Part model, mm, in its own coordinate system. Face numbers are marked on the shaded views. A direction names the side the tool comes from. Coordinates: 2 decimals unless noted, no trailing zeros. Order: outer loops, then holes, each group sorted by start corner. A loop starts at its lowest first (then second) coordinate and runs counter-clockwise, first axis right, second up.
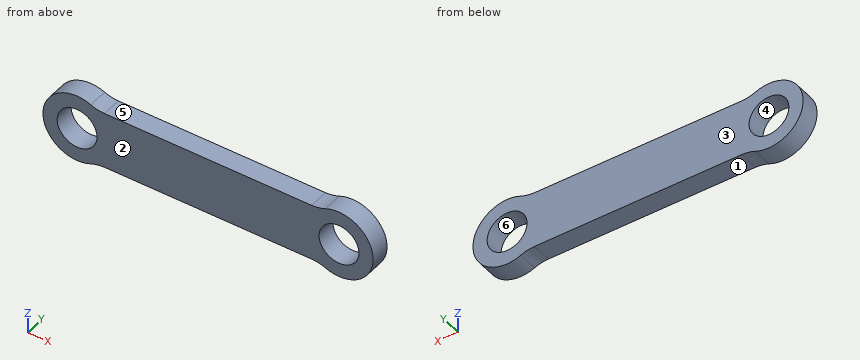
```python
from build123d import *

# Parameters (mm, degrees)
SKETCH1_R           = 1.75
BOSS_EXTRUDE1_DEPTH = 1.75
FILLET1_R           = 3


with BuildPart() as part:
    # Sketch1 → Boss-Extrude1 (new body)
    with BuildSketch(Plane(origin=(0, 0, 0), x_dir=(1, 0, 0), z_dir=(0, 1, 0))):
        with BuildLine():
            ThreePointArc((1.658312395, 2.5), (-3, 0), (1.658312395, -2.5))
            Line((1.658312395, -2.5), (21.341687605, -2.5))
            ThreePointArc((21.341687605, -2.5), (26, 0), (21.341687605, 2.5))
            Line((21.341687605, 2.5), (1.658312395, 2.5))
        make_face()
        with Locations(Location((0, 0, 0), (0, 0, 270))):
            Circle(SKETCH1_R, mode=Mode.SUBTRACT)
        with Locations(Location((23, 0, 0), (0, 0, 270))):
            Circle(SKETCH1_R, mode=Mode.SUBTRACT)
    extrude(amount=BOSS_EXTRUDE1_DEPTH)

    # Fillet1
    fillet1_edges = [part.edges().sort_by_distance(p)[0] for p in [
        (21.341687605, 0.875, 2.5),
        (1.658312395, 0.875, 2.5),
        (1.658312395, 0.875, -2.5),
        (21.341687605, 0.875, -2.5),
    ]]
    fillet(fillet1_edges, radius=FILLET1_R)


solid = part.part
```
(1) Tool access for the marked faces 1 and 2: list every direction of +Z, -Z, +X, -X, +Y, -Y with a clear straight run to the whole face (end or side of a thin tool).
(2) Slice it at D-D, the plane x = 9. Give the cut face in (y, z), then the cut area to 3 significant figures.
(3) Slice it at B-B, the plane y = 1.15. Give the cut face in (x, z).
(4) Slice it at C-C, the plane z = 0. Give the cut face in (x, y).
(5) Slice it at A-A, the plane x = 23. Give the cut face in (y, z).
(6) Probe line 1 (X direction, y = 1.3, z = 0); line 2 (X direction, y = 0.5, z = 1.35); line 3 (Z direction, x = -0.5, y = 0.9). List the from-to ranges inside material, lowest first.
(7) Drop flat-ended pins along their axis: pin 1 (0.5 mm diameter, centred on x = 15.5, y = 1, fed in from -Z); pin 2 (2 mm diameter, centred on x = 0, z = 0, fed in from +Y). Give the stop position or say it passes through.
(8) Pull direction Z, two halves, no side cores. Call the marked faces 3, 4, 5 and 6: +Z half, -Z half, draft (parallel to the pull), parting line (faces both ways), or undercut.
Here are the results:
1. face 1: -Z, +Y, -Y
1. face 2: +Z, -Z, +X, -X, -Y
2. outline: (0, -2.5) - (1.75, -2.5) - (1.75, 2.5) - (0, 2.5) - close
2. area: 8.75 mm2
3. outline: (1.2, -2.75) arc R3 cw to (2.4, -2.5) - (20.6, -2.5) arc R3 cw to (21.8, -2.75) arc R3 ccw (long way) to (21.8, 2.75) arc R3 cw to (20.6, 2.5) - (2.4, 2.5) arc R3 cw to (1.2, 2.75) arc R3 ccw (long way) to start; hole circle Ø3.5 at (0, 0); hole circle Ø3.5 at (23, 0)
4. outline: (-3, 0) - (-1.75, 0) - (-1.75, 1.75) - (-3, 1.75) - close; (1.75, 0) - (21.25, 0) - (21.25, 1.75) - (1.75, 1.75) - close; (24.75, 0) - (26, 0) - (26, 1.75) - (24.75, 1.75) - close
5. outline: (0, -3) - (1.75, -3) - (1.75, -1.75) - (0, -1.75) - close; (0, 1.75) - (1.75, 1.75) - (1.75, 3) - (0, 3) - close
6. line 1: x = -3 to -1.75, 1.75 to 21.25, 24.75 to 26
6. line 2: x = -2.68 to -1.11, 1.11 to 21.89, 24.11 to 25.68
6. line 3: z = -2.96 to -1.68, 1.68 to 2.96
7. pin 1: stops at z = -2.5
7. pin 2: passes through
8. face 3: draft
8. face 4: undercut
8. face 5: +Z half
8. face 6: undercut
